Input: part model. Units: mm. Frame: model coordinates. A direction names the side the tool comes from. Coordinates: 2 decimals unless noted, no trailing zeros. Write each loop counter-clockwise with the first axis right and the second up, starting at its lowest first coordinate (ties: lowest second). Pieces come first, ordered by that corner, then holes. Notation, with made-up numbers: (-1, -3.5) - (17, -3.5) arc R18 cw to (17, 16.5) - close; hole circle Ø7 at (-12, 20). An arc over 180 degrees is marked (long way). Use CSV: the item, a comma, the result in double quotes.
Autodesk Fusion 360 part; units mm, degrees
sketch "Sketch1" plane through (0, 0, 0) normal (0, 0, 1) x (1, 0, 0)
  line L0 (10.5, -4.75) -> (-10.5, -4.75)
  line L1 (-10.5, -4.75) -> (-10.5, 4.75)
  line L2 (-10.5, 4.75) -> (10.5, 4.75)
  line L3 (10.5, 4.75) -> (10.5, -4.75)
  line L4 (10.5, -4.75) -> (-10.5, 4.75) construction
  line L5 (-10.5, -4.75) -> (10.5, 4.75) construction
  dimension "d1" = 21
  dimension "d2" = 9.5
extrude "Extrude1" add sketch "Sketch1" along normal blind 11
sketch "Sketch2" plane through (0, 0, 0) normal (0, 0, -1) x (1, 0, 0)
  line L0 (-10.5, -4.75) -> (10.5, -4.75)
  line L1 (10.5, -4.75) -> (10.5, 4.75)
  line L2 (10.5, 4.75) -> (-10.5, 4.75)
  line L3 (-10.5, 4.75) -> (-10.5, -4.75)
  line L4 (2.05, -0.625) -> (-2.05, -0.625)
  line L5 (-2.05, -0.625) -> (-2.05, 0.625)
  line L6 (-2.05, 0.625) -> (2.05, 0.625)
  line L7 (2.05, 0.625) -> (2.05, -0.625)
  line L8 (2.05, -0.625) -> (-2.05, 0.625) construction
  line L9 (-2.05, -0.625) -> (2.05, 0.625) construction
  dimension "d5" = 4.1
  dimension "d6" = 1.25
sketch "Sketch3" plane through (0, -4.75, 0) normal (0, -1, 0) x (1, 0, 0)
  line L0 (-10.5, 0) -> (10.5, 0)
  line L1 (10.5, 0) -> (10.5, 11)
  line L2 (10.5, 11) -> (-10.5, 11)
  line L3 (-10.5, 11) -> (-10.5, 0)
  spline S0 degree 5 poles (-10.5, 11) (-10.0801, 10.6955) (-9.2404, 10.113) (-7.9808, 9.3191) (-6.3012, 8.4228) (-4.2016, 7.5911) (-2.1018, 7.0739) (-0.0019, 6.8968) (2.0982, 7.0739) (4.1984, 7.5912) (6.2988, 8.4229) (7.9792, 9.3192) (9.2396, 10.1131) (10.0799, 10.6955) (10.5, 11) knots 0 0 0 0 0 0 0.1 0.2 0.3 0.4 0.5 0.6 0.7 0.8 0.9 1 1 1 1 1 1
  line L4 (-0.0031, 6.9851) -> (-0.0336, 6.9851)
  line L5 (-0.5, 7.0404) -> (-0.5, 6.0404)
  line L6 (-0.5, 6.0404) -> (0.5, 6.0404)
  line L7 (0.5, 6.0404) -> (0.5, 6.9951)
  line L8 (0, 11) -> (0, 10) construction
  line L9 (-0.5, 7.0404) -> (-1.1379, 8.2493)
  line L10 (-1.1379, 8.2493) -> (-2.1854, 7.1728)
  line L11 (-2.5306, 7.2364) -> (-3.0769, 8.6476)
  line L12 (-3.0769, 8.6476) -> (-4.3485, 7.7175)
  line L13 (-4.6784, 7.8304) -> (-4.9948, 9.181)
  line L14 (-4.9948, 9.181) -> (-6.3365, 8.5115)
  line L15 (-6.7604, 8.715) -> (-7.1089, 9.9152)
  line L16 (-7.1089, 9.9152) -> (-8.3208, 9.5633)
  line L17 (-8.9482, 9.9473) -> (-8.9482, 11)
  line L18 (0.5, 6.9951) -> (0.5, 7.565)
  line L19 (0.5, 7.0404) -> (1.1379, 8.2493)
  line L20 (1.1379, 8.2493) -> (2.1854, 7.1728)
  line L21 (2.5306, 7.2364) -> (3.0769, 8.6476)
  line L22 (3.0769, 8.6476) -> (4.3485, 7.7175)
  line L23 (4.6784, 7.8304) -> (4.9948, 9.181)
  line L24 (4.9948, 9.181) -> (6.3365, 8.5115)
  line L25 (6.7604, 8.715) -> (7.1089, 9.9152)
  line L26 (7.1089, 9.9152) -> (8.3208, 9.5633)
  line L27 (8.9482, 9.9473) -> (8.9482, 11)
  point P0 (-0.0031, 6.9851)
  dimension "d10" = 0.5
  dimension "d11" = 1
  dimension "d12" = 1
extrude "Extrude2" cut sketch "Sketch2" against normal blind 5 contours L4 L5 L6 L7
extrude "Extrude5" cut sketch "Sketch3" against normal blind 9.5 contours L2 S0 L4 L5 L9 L10 L11 L12 L13 L14 L15 L16 L17 L18 L19 L20 L21 L22 L23 L24 L25 L26 L27 | S0 L4 L5 L6 L7
fillet "Fillet2" radius 0.3 10 edges at (-8.9482, 0, 11) (-7.1089, 0, 9.9152) (-4.9948, 0, 9.181) (-3.0769, 0, 8.6476) (-1.1379, 0, 8.2493) (1.1379, 0, 8.2493) (3.0769, 0, 8.6476) (4.9948, 0, 9.181) (7.1089, 0, 9.9152) (8.9482, 0, 11)
fillet "Fillet3" radius 0.5 2 edges at (10.5, 0, 11) (-10.5, 0, 11)
extrude "Extrude6" add 1 faces at (-7.6833, 0.2083, 0) along direction (0, 0, -1) blind 2
chamfer "Chamfer2" distance 1.5 angle 45 2 edges at (-10.5, 0, -2) (10.5, 0, -2)
(1) Reachability of faces 1 (the flat face through (10.5, 0, 5)), 2 (the flat face through (-4.79, -0.07, 8.31)), 3 (the flat face through (-2.05, 0, 2)) from +Z, -Z, +X, -X, +Y, -Y: full face, straight path, thin tool, end or side. Return the list, or none.
Check values:
face 1,"+Z, -Z, +X, +Y, -Y"
face 2,"+Z, +Y, -Y"
face 3,"-Z"
(2) Cut plane C-C on x = 7.75. Return loops of the section in (y, z), and give its area (3 significant figures).
Check values:
outline,"(-4.75, -2) - (4.75, -2) - (4.75, 9.73) - (-4.75, 9.73) - close"
area,"111 mm^2"
(3) Cut plane A-A on z = -0.25. Return loops of the section in (x, y) (3 decimals).
Check values:
outline,"(-10.5, -4.75) - (10.5, -4.75) - (10.5, 4.75) - (-10.5, 4.75) - close; hole (-2.05, -0.625) - (2.05, -0.625) - (2.05, 0.625) - (-2.05, 0.625) - close"
(4) Draft query along X for faces 4 (the flat face through (0, -4.75, 3)), 5 (the flat face through (-0.5, -0.1, 6.5)), 6 (the flat face through (-10.5, 0, 5)). Return one class per face: pulls with the +X half, pulls with the -X half, needs draft (parallel to the pull), parting line crosses it, or undercut.
Check values:
face 4,"needs draft"
face 5,"undercut"
face 6,"pulls with the -X half"
(5) Cut plane B-B on x = 1.75. Return loops of the section in (y, z) (3 decimals).
Check values:
outline,"(-4.75, -2) - (-0.625, -2) - (-0.625, 5) - (0.625, 5) - (0.625, -2) - (4.75, -2) - (4.75, 7.62) - (-4.75, 7.62) - close"
(6) Ray query, probe 1 along Y at (x, z) = (1, -0.75) (3 decimals); probe 2 along X at (y, z) = (-2.5, 7); probe 3 along Z at (x, y) = (-1, 0.5). Return the intervals inside material, ascending. Write a range as from..to.
Check values:
probe 1,"-4.75..-0.625, 0.625..4.75"
probe 2,"-10.5..-0.5, 0.5..10.5"
probe 3,"5..7.96"
(7) Pin query (flat end, axial travel): pin 1 Ø4 at (x, y) = (-2.5, 1) entering from +Z; pin 2 Ø1 at (x, y) = (0.5, 0) entering from -Z; pin 3 Ø1.1 at (x, y) = (0, 0) entering from +Z. Return the tip coordinate at first contact, or that it passes through.
Check values:
pin 1,"z = 8.47"
pin 2,"z = 5"
pin 3,"z = 7.14"
